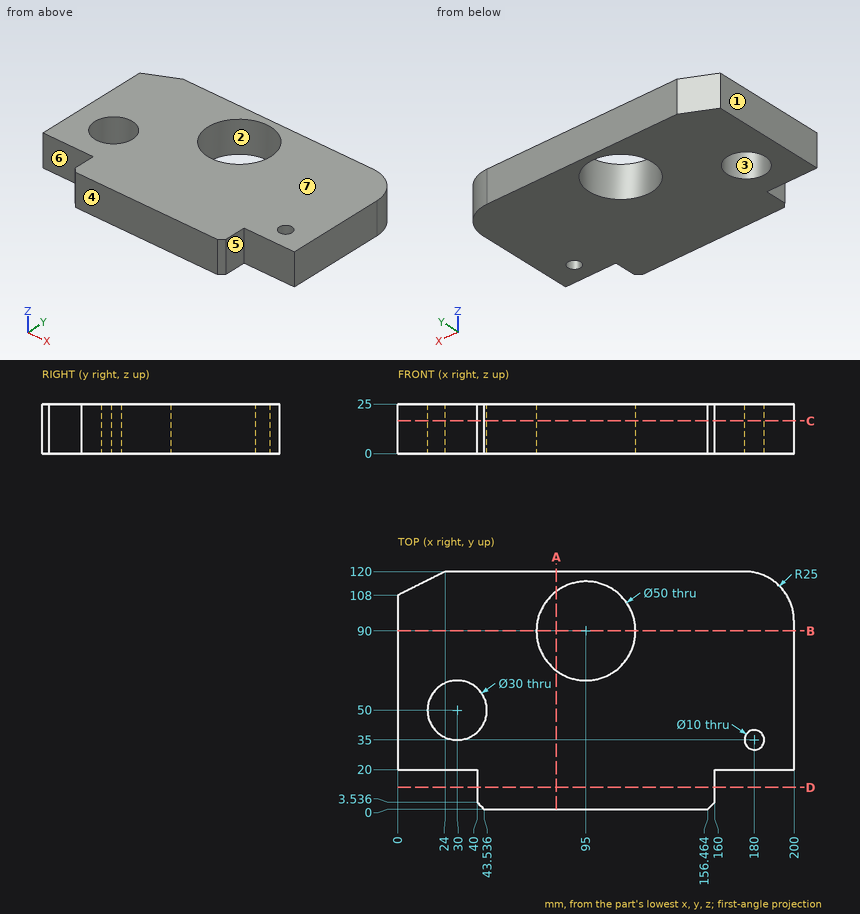
Could you check a few things on this drawing? It's one solid part, dimensions in mm from its lowest x, y, z. A direction names the side the tool comes from. Round coordinates to 2 decimals unless told otherwise and drop trailing zeros. Write each loop counter-clockwise with the first axis right and the second up, starting at its lowest first coordinate (ties: lowest second). Pieces come first, ordered by that corner, then holes. Notation, with made-up numbers: (71.25, 25) -> (121.25, 25) arc R26 ccw to (121.25, 46) -> close; hole circle Ø5 at (87, 2). An arc over 180 degrees is marked (long way). Use one line per item in the form item = value. Start each with the question number.
Q1. Imagine slicing it at B-B (y = 90). Please give me the cut outline in (x, z), then the cut area to 3 significant figures.
Q2. Imagine slicing it at C-C (z = 16.5). Please give me the cut outline in (x, y) (1 decimal), then the cut area to 3 significant figures.
Q3. We'd pull the mould along Y, two halves only. Please class the marked faces 1, 2, 3 and 4: +Y half, -Y half, draft (parallel to the pull), parting line (faces both ways), or undercut.
Q4. Imagine slicing it at A-A (x = 80). Please give me the cut outline in (y, z), then the cut area to 3 significant figures.
Q5. If I drill on probe 1 along X at (y, z) = (34.5, 1.75) (1 decimal); probe 2 along Y at (x, z) = (96, 12.5); probe 3 along X at (y, z) = (18.5, 15), over which ranges is the centre line in solid material (lowest first)? Write a range as [from, to].
Q6. Which directions (+Z, -Z, +X, -X, +Y, -Y) give clear straight access to the entire face, cutting with the end or side of a thin tool? Please do the marked faces 5, 6 and 7.
Q7. Imagine slicing it at D-D (y = 11). Please give me the cut outline in (x, z).
Q8. I'm going to push flat-ended pins straight in: P1, Ø12, axis at y = 50.5, z = 11, coming from the -X side; P2, Ø12.5, axis at x = 12.5, z = 7.5, coming from the -Y side; P3, Ø8, axis at y = 8, z = 15.5, coming from the -X side; P4, Ø10, axis at x = 37.5, z = 5.5, coming from the -Y side (1 decimal). Where does each tip first touch, or does it pass through?
Worked out:
q1.outline = (0, 0) -> (70, 0) -> (70, 25) -> (0, 25) -> close; (120, 0) -> (200, 0) -> (200, 25) -> (120, 25) -> close
q1.area = 3,750 mm^2
q2.outline = (0, 20) -> (40, 20) -> (40, 3.5) -> (43.5, 0) -> (156.5, 0) -> (160, 3.5) -> (160, 20) -> (200, 20) -> (200, 95) arc R25 ccw to (175, 120) -> (24, 120) -> (0, 108) -> close; hole circle Ø30 at (30, 50); hole circle Ø50 at (95, 90); hole circle Ø10 at (180, 35)
q2.area = 19,400 mm^2
q3.face_1 = draft
q3.face_2 = undercut
q3.face_3 = undercut
q3.face_4 = -Y half
q4.outline = (0, 0) -> (70, 0) -> (70, 25) -> (0, 25) -> close; (110, 0) -> (120, 0) -> (120, 25) -> (110, 25) -> close
q4.area = 2,000 mm^2
q5.probe_1 = [0, 175], [185, 200]
q5.probe_2 = [0, 65.02], [114.98, 120]
q5.probe_3 = [40, 160]
q6.face_5 = +Z, -Z, +X, -Y
q6.face_6 = +Z, -Z, -X, -Y
q6.face_7 = +Z, +X, -X, +Y, -Y
q7.outline = (40, 0) -> (160, 0) -> (160, 25) -> (40, 25) -> close
q8.P1 = 0
q8.P2 = 20
q8.P3 = 40
q8.P4 = 1
